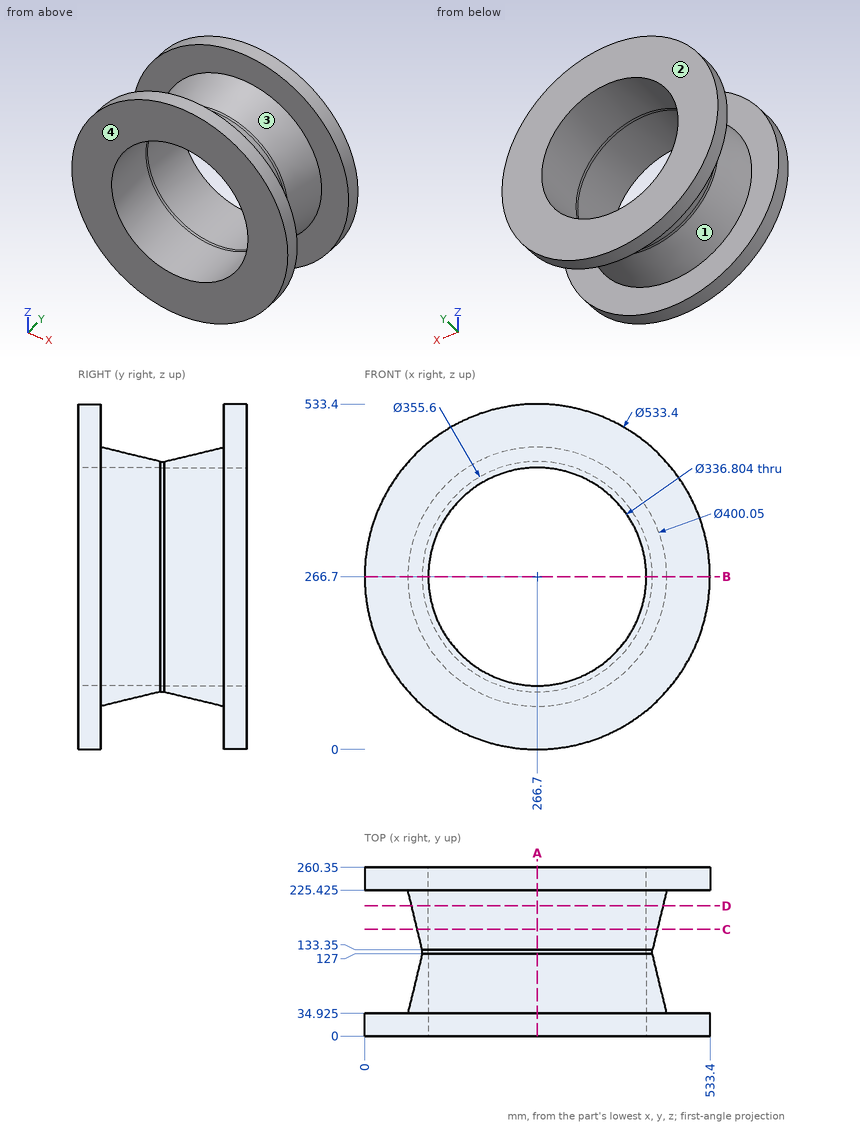
Study the drawing (mm; zero at the part's minimum x, y, z) and answer. Give positions to 0.01 mm unless a question says otherwise; leave off trailing zeros. Loops run counter-clockwise (first coordinate to the right, second up) from the corner with the lowest first, then second, coordinate; pieces in that order, holes last. Notation, with made-up numbers: M -11,58 L 40,58 A28 ccw 40,95 Z; hole C 82.5,52 d9. An arc over 180 degrees is marked long. One line per item, written item: value.
1. Section B-B on z = 266.7 is taken. Determine the outline of the cut face in (x, y) (3 decimals).
Found:
outline: M 0,0 L 98.298,0 L 98.298,260.35 L 0,260.35 L 0,225.425 L 66.675,225.425 L 88.9,133.35 L 88.9,127 L 66.675,34.925 L 0,34.925 Z; M 435.102,0 L 533.4,0 L 533.4,34.925 L 466.725,34.925 L 444.5,127 L 444.5,133.35 L 466.725,225.425 L 533.4,225.425 L 533.4,260.35 L 435.102,260.35 Z
2. Section A-A on x = 266.7 is taken. Determine the outline of the cut face in (y, z) (3 decimals).
Found:
outline: M 0,0 L 34.925,0 L 34.925,66.675 L 127,88.9 L 133.35,88.9 L 225.425,66.675 L 225.425,0 L 260.35,0 L 260.35,98.298 L 0,98.298 Z; M 0,435.102 L 260.35,435.102 L 260.35,533.4 L 225.425,533.4 L 225.425,466.725 L 133.35,444.5 L 127,444.5 L 34.925,466.725 L 34.925,533.4 L 0,533.4 Z
3. Section D-D on y = 201 is taken. Determine the outline of the cut face in (x, z), plus the area to 3 significant figures.
Found:
outline: C 266.7,266.7 d388.26; hole C 266.7,266.7 d336.8
area: 29,300 mm^2
4. Each of these flat-tipped pins is pushed along its axis until it touches: P1, Ø5, axis at x = 479.5, z = 402, coming from the -Y side; P2, Ø3, axis at x = 149.5, y = 218, coming from the -Z side; P3, Ø3, axis at x = 314.5, y = 111, coming from the -Z side; P4, Ø4, axis at x = 255, y = 217.5, coming from the +Z side. Where does it stop, or does it pass through?
Found:
P1: y = 0
P2: z = 105.65
P3: z = 90.89
P4: z = 464.96
5. For a pull along Y with two mould halves and no side action, classify the marked faces 1, 2, 3 and 4 as pulls with the +Y half, pulls with the -Y half, needs draft (parallel to the pull), parting line crosses it, or undercut.
Found:
face 1: undercut
face 2: pulls with the +Y half
face 3: undercut
face 4: pulls with the -Y half
6. Section C-C on y = 164.5 is taken. Determine the outline of the cut face in (x, z).
Found:
outline: C 266.7,266.7 d370.64; hole C 266.7,266.7 d336.8
7. Find the intervals of material crossed by probe 1 along Y at (x, z) = (98, 107.5) (3 decimals); probe 2 along Z at (x, y) = (266, 131); probe 3 along X at (y, z) = (225, 266), in increasing order.
Found:
probe 1: 0 to 34.925, 225.425 to 260.35
probe 2: 88.9 to 98.3, 435.1 to 444.5
probe 3: 66.78 to 98.3, 435.1 to 466.62
